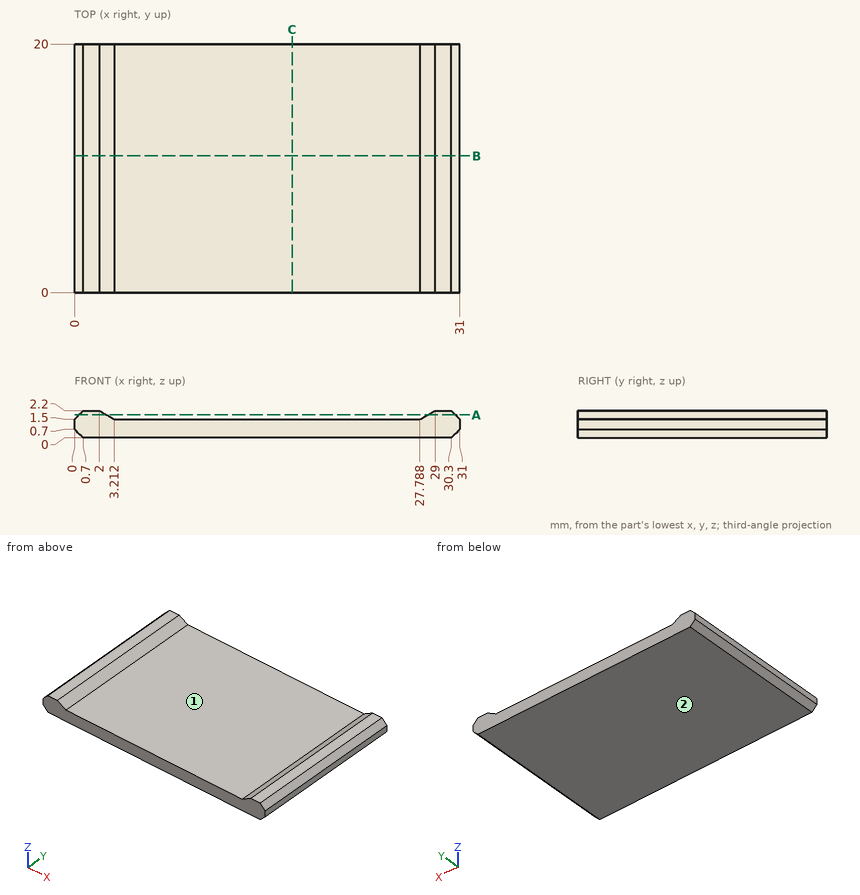
Check sheet for the drawn part. Datum: minimum x, y, z corner. Units: mm. Give positions to 0.01 mm unless a question says otherwise; leave off trailing zeros. Write each loop counter-clockwise with the first axis right and the second up, starting at its lowest first coordinate (ties: lowest second). Pieces come first, ordered by that corner, then holes. Notation, with made-up numbers: (51.5, 27) -> (74.5, 27) arc R16 cw to (74.5, 37) -> close; hole circle Ø1 at (73.25, 84). An arc over 180 degrees is marked (long way). Use one line per item in the form item = value. Start each with the question number.
1. Section check A-A (z = 1.85). Record the cut outline in (x, y).
2. Mould release check, pull along X, two halves, no side actions. Record for the marked faces 1 and 2: pulls with the +X half, pulls with the -X half, needs draft (parallel to the pull), parting line crosses it, or undercut.
3. Go/stop test with a flat-tipped pin: P1, Ø4, axis at x = 17, y = 7, coming from the +Z side. Record where the tip stops, or that it passes through.
4. Section check B-B (y = 11). Record the cut outline in (x, z).
5. Thickness scan on line 1 along Z through (x, y) = (8, 14.5); line 2 along X through (y, z) = (5.25, 2.1) (1 decimal); line 3 along Z through (x, y) = (3, 12.5). Record the ranges inside material, lowest first. Write a range as from..to.
6. Section check C-C (x = 17.5). Record the cut outline in (y, z).
Conclusion:
q1.outline = (0.35, 0) -> (2.61, 0) -> (2.61, 20) -> (0.35, 20) -> close; (28.39, 0) -> (30.65, 0) -> (30.65, 20) -> (28.39, 20) -> close
q2.face_1 = undercut
q2.face_2 = needs draft
q3.P1 = 1.5
q4.outline = (0, 0.7) -> (0.7, 0) -> (30.3, 0) -> (31, 0.7) -> (31, 1.5) -> (30.3, 2.2) -> (29, 2.2) -> (27.79, 1.5) -> (3.21, 1.5) -> (2, 2.2) -> (0.7, 2.2) -> (0, 1.5) -> close
q5.line_1 = 0..1.5
q5.line_2 = 0.6..2.2, 28.8..30.4
q5.line_3 = 0..1.62
q6.outline = (0, 0) -> (20, 0) -> (20, 1.5) -> (0, 1.5) -> close
